Work out the finished part from the listing and answer in its coordinate system (mm). Coordinates: 2 decimals unless noted, no trailing zeros. Loops run counter-clockwise (first coordinate to the right, second up) from the corner with the lowest first, then second, coordinate; pieces in that order, holes last. Notation, with made-up numbers: (50, 62) - (55, 62) arc R21 ccw to (55, 75) - close; hole circle Ø7 at (-35, -25). An arc over 180 degrees is marked (long way). Write each question's results on one line, items separated by ' | '. Start each with the question number.
1. A cutting plane is placed at D-D on x = 82. Determine the outline of the cut face in (y, z).
2. Find the intervals of material crossed by line 1 along Y through (x, z) = (126.16, 1); line 2 along Y through (x, z) = (127, 1.65); line 3 along Y through (x, z) = (-21, 1.55), in increasing order. Write a range as [from, to].
3. A cutting plane is placed at A-A on x = 150.16. Determine the outline of the cut face in (y, z), then the cut area to 3 significant figures.
4. A cutting plane is placed at C-C on z = 1.65. State how many separate pieces and enclosed holes the cut face has, then the cut area to 3 significant figures.
5. Each of these flat-tipped pins is pushed along its axis until it touches: P1, Ø4.5, axis at x = -20, y = 159.597, coming from the +Z side; P2, Ø1.5, axis at x = -4, z = 2.5, coming from the -Y side; P3, Ø1, axis at y = 89.5, z = 1, coming from the +X side. Where does it stop, or does it pass through?
6. A cutting plane is placed at B-B on y = 55. Determine the outline of the cut face in (x, z), then the cut area to 3 significant figures.
Autodesk Inventor part; units mm, degrees
ref_plane "YZ Plane" through (0, 0, 0) normal (1, 0, 0) x (0, 1, 0)
ref_plane "XZ Plane" through (0, 0, 0) normal (0, 1, 0) x (-1, 0, 0)
ref_plane "XY Plane" through (0, 0, 0) normal (0, 0, 1) x (1, 0, 0)
sketch "スケッチ1" plane through (0, 0, 0) normal (0, 0, 1) x (1, 0, 0)
  line L0 (0, 0) -> (130.16, 0)
  line L1 (130.16, 0) -> (130.16, 159.597)
  line L2 (130.16, 159.597) -> (0, 159.597)
  line L3 (0, 159.597) -> (0, 0)
  dimension "d0" = 130.16
  dimension "d1" = 159.597
extrude "押し出し1" add sketch "スケッチ1" along normal blind 3
sketch "スケッチ2" plane through (0, 0, 3) normal (0, 0, 1) x (1, 0, 0)
  line L0 (126.16, 3.92) -> (126.16, 113.08) construction
  circle A0 centre (126.16, 3.92) radius 1.6
  circle A1 centre (126.16, 113.08) radius 1.6
  line L1 (130.16, 0) -> (130.16, 159.597)
  line L2 (0, 0) -> (130.16, 0)
  circle A2 centre (121.531, 154.597) radius 1.6
  line L3 (130.16, 159.597) -> (0, 159.597)
  line L4 (121.531, 154.597) -> (121.531, 139.097) construction
  circle A3 centre (121.531, 139.097) radius 1.6
  line L5 (18.398, 154.597) -> (33.898, 154.597) construction
  line L6 (0, 159.597) -> (0, 0) construction
  circle A4 centre (18.398, 154.597) radius 1.6
  circle A5 centre (33.898, 154.597) radius 1.6
  dimension "d4" = 3.2
  dimension "d5" = 4
  dimension "d6" = 3.92
  dimension "d7" = 109.16
  dimension "d10" = 5
  dimension "d11" = 8.629
  dimension "d12" = 15.5
  dimension "d13" = 18.398
  dimension "d14" = 5
  dimension "d15" = 15.5
extrude "押し出し2" cut sketch "スケッチ2" against normal blind 3
sketch "スケッチ4" plane through (0, 0, 3) normal (0, 0, 1) x (1, 0, 0)
  line L0 (130.16, 159.597) -> (0, 159.597) construction
  line L1 (130.16, 0) -> (130.16, 159.597) construction
  line L2 (0, 159.597) -> (0, 0) construction
  line L3 (0, 159.597) -> (-30, 159.597)
  line L4 (-30, 159.597) -> (-30, 129.597)
  line L5 (-30, 129.597) -> (0, 129.597)
  line L6 (0, 129.597) -> (0, 159.597)
  line L7 (130.16, 159.597) -> (160.16, 159.597)
  line L8 (160.16, 159.597) -> (160.16, 129.597)
  line L9 (160.16, 129.597) -> (130.16, 129.597)
  line L10 (130.16, 129.597) -> (130.16, 159.597)
  circle A0 centre (-20, 149.597) radius 2.75
  circle A1 centre (150.16, 149.597) radius 2.75
  dimension "d23" = 30
  dimension "d24" = 30
  dimension "d26" = 10
  dimension "d27" = 10
  dimension "d28" = 10
  dimension "d29" = 10
  dimension "d30" = 5.5
extrude "押し出し4" add sketch "スケッチ4" against normal blind 3
sketch "スケッチ3" plane through (0, 0, 3) normal (0, 0, 1) x (1, 0, 0)
  circle A0 centre (55.16, 89.597) radius 30 construction
  line L0 (0, 159.597) -> (0, 0) construction
  line L1 (0, 129.597) -> (60.2796, 119.1569)
  line L2 (84.9814, 92.8656) -> (95.16, 0)
  line L3 (0, 0) -> (130.16, 0) construction
  line L4 (130.16, 159.597) -> (0, 159.597) construction
  line L5 (130.16, 0) -> (130.16, 159.597) construction
  arc A1 (84.9814, 92.8656) -> (60.2796, 119.1569) centre (55.16, 89.597) ccw
  line L6 (0, 129.597) -> (0, 0)
  line L7 (0, 0) -> (95.16, 0)
  dimension "d16" = 30
  dimension "d17" = 35
  dimension "d18" = 70
  dimension "d19" = 75
  dimension "d20" = 60
extrude "押し出し3" cut sketch "スケッチ3" against normal blind 3
sketch "スケッチ5" plane through (0, 0, 3) normal (0, 0, 1) x (1, 0, 0)
  line L0 (-30, 159.597) -> (160.16, 159.597) construction
  line L1 (65.08, 159.597) -> (65.08, 0) construction
  line L2 (0, 129.597) -> (60.2796, 119.1569) construction
  line L3 (0, 129.597) -> (-30, 134.7928)
  line L4 (-30, 134.7928) -> (-30, 129.597)
  line L5 (-30, 129.597) -> (0, 129.597)
  line L6 (130.16, 129.597) -> (160.16, 134.7928)
  line L7 (160.16, 134.7928) -> (160.16, 129.597)
  line L8 (160.16, 129.597) -> (130.16, 129.597)
  point P0 (0, 0)
extrude "押し出し5" cut sketch "スケッチ5" against normal blind 3
fillet "フィレット1" radius 30 1 edges at (130.16, 129.597, 1.5)
sketch "スケッチ6" plane through (0, 0, 3) normal (0, 0, 1) x (1, 0, 0)
  line L0 (-30, 159.597) -> (160.16, 159.597) construction
  line L1 (-30, 159.597) -> (-30, 134.7928)
  line L2 (-30, 159.597) -> (160.16, 159.597)
  line L3 (160.16, 159.597) -> (160.16, 169.597)
  line L4 (160.16, 169.597) -> (-30, 169.597)
  line L5 (-30, 169.597) -> (-30, 159.597)
  line L6 (160.16, 159.597) -> (160.16, 134.7928)
  point P0 (0, 0)
  dimension "d38" = 10
extrude "押し出し6" add sketch "スケッチ6" against normal blind 3
sketch "スケッチ7" plane through (0, 0, 3) normal (0, 0, 1) x (1, 0, 0)
  circle A0 centre (-20, 149.597) radius 2.75 construction
  circle A1 centre (150.16, 149.597) radius 2.75 construction
  line L0 (-20, 149.597) -> (-20, 159.597) construction
  circle A2 centre (-20, 159.597) radius 2.75
  line L1 (150.16, 149.597) -> (150.16, 159.597) construction
  circle A3 centre (150.16, 159.597) radius 2.75
  point P0 (0, 0)
  dimension "d41" = 10
extrude "押し出し7" cut sketch "スケッチ7" against normal blind 3
sketch "スケッチ8" plane through (0, 0, 3) normal (0, 0, 1) x (1, 0, 0)
  circle A0 centre (-20, 149.597) radius 2.75
  circle A1 centre (150.16, 149.597) radius 2.75
  point P0 (0, 0)
extrude "押し出し8" add sketch "スケッチ8" against normal blind 3
fillet "フィレット2" radius 10 3 edges at (-30, 134.7928, 1.5) (160.16, 134.7928, 1.5) (95.16, 0, 1.5)
fillet "フィレット2" radius 2 1 edges at (130.16, 0, 1.5)
sketch "スケッチ9" plane through (0, 0, 3) normal (0, 0, 1) x (1, 0, 0)
  line L0 (160.16, 169.597) -> (-30, 169.597)
  line L1 (160.16, 143.076) -> (160.16, 169.597)
  line L2 (-30, 169.597) -> (160.16, 169.597)
  line L3 (160.16, 169.597) -> (160.16, 169.097)
  line L4 (160.16, 169.097) -> (-30, 169.097)
  line L5 (-30, 169.097) -> (-30, 169.597)
  point P0 (0, 0)
  dimension "d46" = 0.5
extrude "押し出し9" cut sketch "スケッチ9" against normal blind 3
fillet "フィレット3" radius 2 2 edges at (-30, 169.097, 1.5) (160.16, 169.097, 1.5)
equation "\"d28\" = d26"
equation "\"d29\" = d27"
properties part number "small_gpu_04" material "アルミニウム 6061"
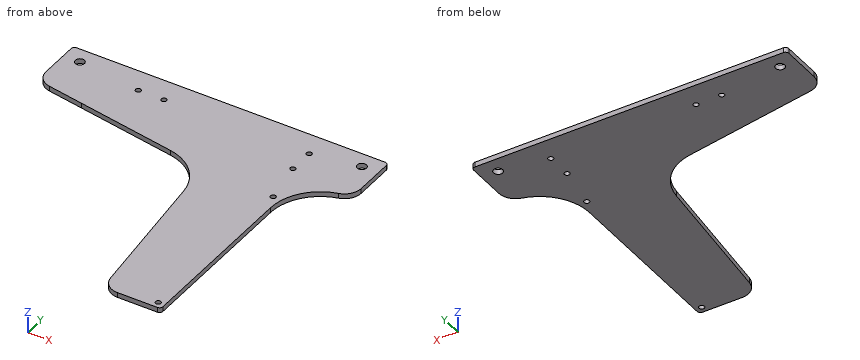
Values:
1) outline: (103, 0) - (169.1, 0) - (169.1, 3) - (103, 3) - close
2) line 1: [0, 2.32], [5.52, 111.48], [114.68, 169.1] | line 2: [0, 2.56], [5.28, 111.72], [114.44, 169.1] | line 3: [133.23, 157.04], [162.16, 169.1]
3) outline: (132.63, 0) - (156.85, 0) - (156.85, 3) - (132.63, 3) - close; (162.35, 0) - (169.1, 0) - (169.1, 3) - (162.35, 3) - close | area: 92.9 mm^2
4) separate pieces: 1 | enclosed holes: 8 | area: 13,500 mm^2
5) P1: through | P2: y = 130.16 | P3: x = 130.16
6) outline: (89.13, 0) - (130.16, 0) - (130.16, 3) - (89.13, 3) - close | area: 123 mm^2
